from build123d import *

# Parameters (mm, degrees)
BOSS_EXTRUDE1_DEPTH      = 18
M3_CLEARANCE_HOLE1_D     = 3.4
M3_CLEARANCE_HOLE1_DEPTH = 12
M3_CLEARANCE_HOLE1_TIP   = 1.021463052
SKETCH5_R                = 1.5
BOSS_EXTRUDE2_DEPTH      = 8


with BuildPart() as part:
    # Sketch1 → Boss-Extrude1 (new body)
    with BuildSketch(Plane(origin=(0, 0, 0), x_dir=(1, 0, 0), z_dir=(0, 1, 0))):
        Polygon((3.175426481, 0), (1.58771324, 2.75), (-1.58771324, 2.75), (-3.175426481, 0), (-1.58771324, -2.75), (1.58771324, -2.75), align=None)
    extrude(amount=BOSS_EXTRUDE1_DEPTH)

    # M3 Clearance Hole1
    with Locations(Plane(origin=(0, 18, 0), x_dir=(-1, 0, 0), z_dir=(0, 1, 0))):
        with Locations((0, 0)):
            Hole(M3_CLEARANCE_HOLE1_D / 2, depth=M3_CLEARANCE_HOLE1_DEPTH)
            with Locations((0, 0, -(M3_CLEARANCE_HOLE1_DEPTH + M3_CLEARANCE_HOLE1_TIP / 2))):  # 118° drill point
                Cone(0, M3_CLEARANCE_HOLE1_D / 2, M3_CLEARANCE_HOLE1_TIP, mode=Mode.SUBTRACT)

    # Sketch4 → Cut-Revolve1 (revolve, cut)
    with BuildSketch(Plane.XY):
        with BuildLine():
            Line((-2.175426481, 18), (-3.175426481, 18))
            Line((-3.175426481, 18), (-3.175426481, 17))
            ThreePointArc((-3.175426481, 17), (-2.882533262, 17.707106781), (-2.175426481, 18))
        make_face()
        with BuildLine():
            Line((-3.175426481, 1), (-3.175426481, 0))
            Line((-3.175426481, 0), (-2.175426481, 0))
            ThreePointArc((-2.175426481, 0), (-2.882533262, 0.292893219), (-3.175426481, 1))
        make_face()
    revolve(axis=Axis((0, 18, 0), (0, -1, 0)), mode=Mode.SUBTRACT)

    # Sketch5 → Boss-Extrude2 (add)
    with BuildSketch(Plane.XZ):
        Circle(SKETCH5_R)
    extrude(amount=BOSS_EXTRUDE2_DEPTH)


solid = part.part
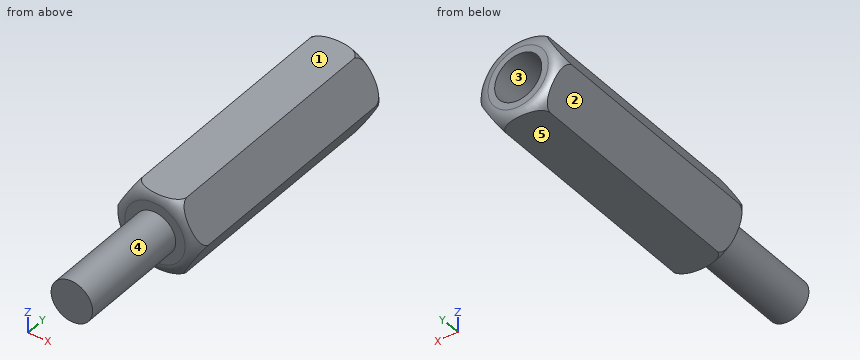
The model under review builds one solid part; all positions refer to its coordinate system, in mm. Face numbers are marked on the shaded views. A direction names the side the tool comes from. Round coordinates to 2 decimals unless told otherwise and drop trailing zeros. Write each loop counter-clockwise with the first axis right and the second up, starting at its lowest first coordinate (ties: lowest second). Pieces come first, ordered by that corner, then holes. Notation, with made-up numbers: M 56.25,-26.5 L 61.25,-26.5 A16 ccw 61.25,4.5 Z; hole C -17,38.25 d7. An arc over 180 degrees is marked long. Answer as CSV lines item,"result". Start each with the question number.
Q1. The part is to be moulded in two halves that separate along Z. For the marked faces 1, 2 and 3, say which applies: +Z half, -Z half, draft (parallel to the pull), parting line (faces both ways), or undercut.
Q2. Consider section A-A, the plane y = 11.75. Give the boundary of the cut face in (x, z), then the cut area to 3 significant figures.
Q3. Wall thickness on line 1 along Z through (x, y) = (0, 12); line 2 along X through (y, z) = (12.5, -0.05); line 3 along Y through (x, z) = (-2, 0.05): over which ranges is each line inside the solid? List them lowest first.
Q4. Consider section B-B, the plane y = 5.5. Give the boundary of the cut face in (x, z), then the cut area to 3 significant figures.
Q5. Tool access review of the marked faces 4 and 5: name each direction out of +Z, -Z, +X, -X, +Y, -Y from which nothing blocks a thin tool from reaching the whole face with its end or side.
Result set:
1,face 1,"+Z half"
1,face 2,"-Z half"
1,face 3,"undercut"
2,outline,"M -3.18,0 L -1.59,-2.75 L 1.59,-2.75 L 3.18,0 L 1.59,2.75 L -1.59,2.75 Z; hole C 0,0 d3.4"
2,area,"17.1 mm²"
3,line 1,"z = -2.75 to -1.7, 1.7 to 2.75"
3,line 2,"x = -3.15 to -1.7, 1.7 to 3.15"
3,line 3,"y = 0 to 18"
4,outline,"M -3.18,0 L -1.59,-2.75 L 1.59,-2.75 L 3.18,0 L 1.59,2.75 L -1.59,2.75 Z; hole C 0,0 d1.74"
4,area,"23.8 mm²"
5,face 4,"-Y"
5,face 5,"-Z, +X, -X, +Y, -Y"
